CAD build for the part. Positions are in the model's coordinates, mm. Round coordinates to 2 decimals unless told otherwise and drop trailing zeros. Order: outer loops, then holes, each group sorted by start corner. A loop starts at its lowest first (then second) coordinate and runs counter-clockwise, first axis right, second up. Notation, with made-up numbers: M 6,-21 L 39,-21 A27 ccw 39,12 Z; hole C 24.5,60.5 d8. An arc over 180 degrees is marked long. Answer as CSV lines item,"result". Start each with the question number.
Autodesk Inventor part; units mm, degrees
ref_plane "YZ Plane" through (0, 0, 0) normal (1, 0, 0) x (0, 1, 0)
ref_plane "XZ Plane" through (0, 0, 0) normal (0, 1, 0) x (-1, 0, 0)
ref_plane "XY Plane" through (0, 0, 0) normal (0, 0, 1) x (1, 0, 0)
sketch "Sketch1" plane through (0, 0, 0) normal (0, 0, 1) x (1, 0, 0)
  line L0 (0, 150.5) -> (7.5, 150.5) construction
  line L1 (15, 150.5) -> (15, -150.5)
  line L2 (15, -150.5) -> (7.5, -150.5)
  line L3 (0, -150.5) -> (0, 150.5)
  line L4 (0, 150.5) -> (7.5, 150.5) construction
  line L5 (7.5, 150.5) -> (7.5, 154.5)
  line L6 (7.5, 154.5) -> (0, 154.5)
  line L7 (0, 154.5) -> (0, 150.5)
  line L8 (0, -150.5) -> (7.5, -150.5) construction
  line L9 (7.5, -150.5) -> (7.5, -154.5)
  line L10 (7.5, -154.5) -> (0, -154.5)
  line L11 (0, -154.5) -> (0, -150.5)
  line L12 (7.5, -150.5) -> (0, -150.5) construction
  line L13 (7.5, 150.5) -> (15, 150.5)
  circle A0 centre (15, 96.116) radius 5.5796
  circle A1 centre (15, -96.116) radius 5.5796
  line L14 (-4.1159, 0) -> (24.6955, 0) construction
  point P0 (0, 0)
  point P1 (0, 0)
  point P2 (3.75, 150.5)
  point P3 (0, 0)
  point P4 (15, -101.6955)
  point P5 (15, -90.5364)
  point P6 (15, 90.5364)
  point P7 (15, 101.6955)
  dimension "d0" = 301
  dimension "d1" = 15
  dimension "d2" = 4
  dimension "d3" = 7.5
  dimension "d4" = 4
  dimension "d5" = 7.5
  dimension "d6" = 150.5
extrude "Extrusion1" add sketch "Sketch1" along normal blind 4 contours L1 A0 A1 L2 L9 L10 L11 L3 L7 L6 L5 L13
properties part number "ReedRail" material "Wood (Oak)"
Q1. Probe line 1 along Y through (x, z) = (10.5, 3.5); line 2 along Y through (x, z) = (11, 2.45); line 3 along Y through (x, z) = (9, 2.2). List the from-to ranges inside material, lowest first. Write a range as from..to.
Q2. Mould opens along Y. For faces 1 (the flat face through (7, 2, 4)), 2 (the cylindrical face through (9.42, 95.99, 1.97)) say: +Y half, -Y half, draft (parallel to the pull), parting line (faces both ways), or undercut.
Q3. Band-saw the part on A-A, the plane x = 12.25. Write the cut outline in (y, z), then the cut area to 3 significant figures.
Q4. Band-saw the part on B-B, the plane z = 0.9. Write the cut outline in (x, y), then the cut area to 3 significant figures.
Answer:
1,line 1,"y = -150.5..-99.41, -92.82..92.82, 99.41..150.5"
1,line 2,"y = -150.5..-100.01, -92.23..92.23, 100.01..150.5"
1,line 3,"y = -150.5..150.5"
2,face 1,"draft"
2,face 2,"undercut"
3,outline,"M -150.5,0 L -100.97,0 L -100.97,4 L -150.5,4 Z; M -91.26,0 L 91.26,0 L 91.26,4 L -91.26,4 Z; M 100.97,0 L 150.5,0 L 150.5,4 L 100.97,4 Z"
3,area,"1,130 mm^2"
4,outline,"M 0,-154.5 L 7.5,-154.5 L 7.5,-150.5 L 15,-150.5 L 15,-101.7 A5.58 cw 15,-90.54 L 15,90.54 A5.58 cw 15,101.7 L 15,150.5 L 7.5,150.5 L 7.5,154.5 L 0,154.5 Z"
4,area,"4,480 mm^2"
